Geometry check sheet. Reference: drawing and pictorial views, mm from the part's lowest x, y, z. Give positions to 0.01 mm unless a question says otherwise; leave off trailing zeros. Order: outer loops, then holes, each group sorted by start corner. A loop starts at its lowest first (then second) coordinate and runs counter-clockwise, first axis right, second up. Notation, with made-up numbers: (89.25, 88.5) -> (126.25, 88.5) arc R7 ccw to (126.25, 99.5) -> close; hole circle Ø5 at (-12, 81.5). An arc over 180 degrees is marked (long way). Write each question's results on one line, items separated by ' | '.
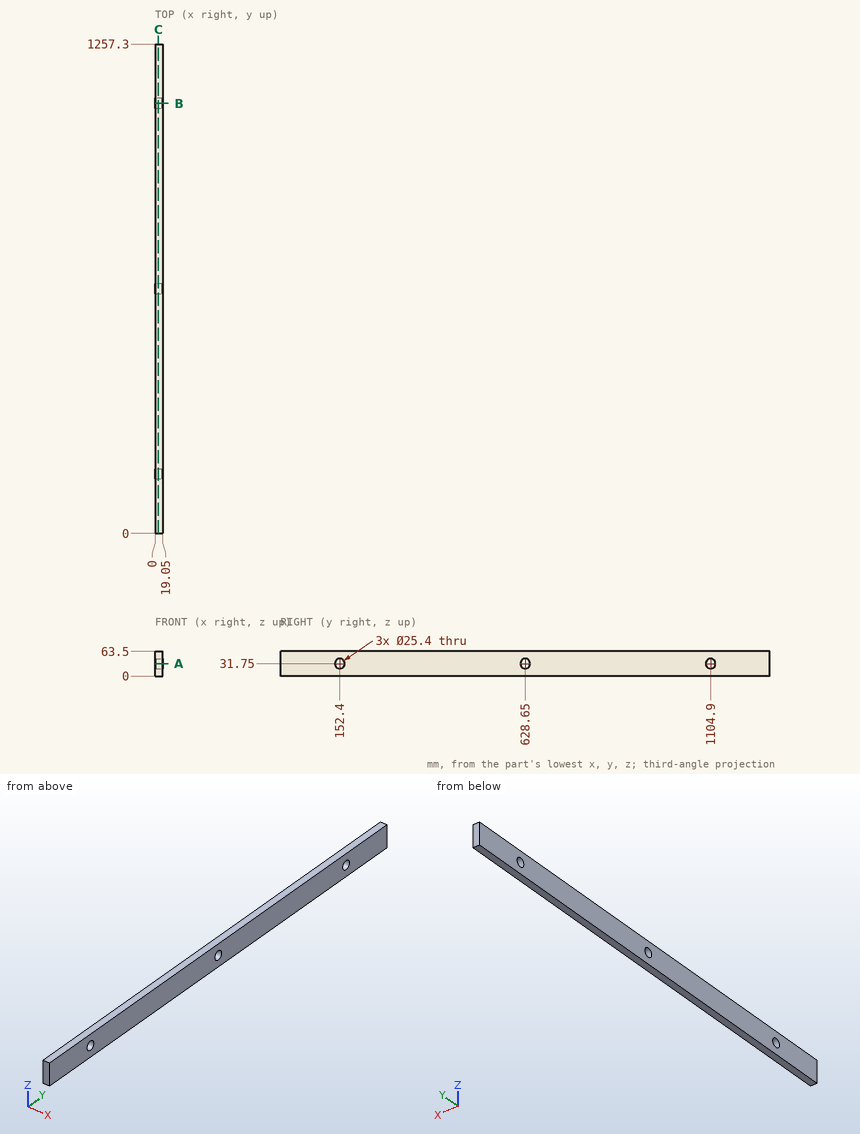
1. Material ranges on probe 1 along Z at (x, y) = (12.5, 628.65); probe 2 along Y at (x, z) = (10.25, 42); probe 3 along Y at (x, z) = (10.25, 43), recorded low to high. Write a range as from..to.
Verdict:
probe 1: z = 0..19.05, 44.45..63.5 | probe 2: y = 0..144.9, 159.9..621.15, 636.15..1097.4, 1112.4..1257.3 | probe 3: y = 0..146.51, 158.29..622.76, 634.54..1099.01, 1110.79..1257.3
2. Section check A-A on z = 31.75. Record the cut outline in (x, y).
Verdict:
outline: (0, 0) -> (19.05, 0) -> (19.05, 139.7) -> (0, 139.7) -> close; (0, 165.1) -> (19.05, 165.1) -> (19.05, 615.95) -> (0, 615.95) -> close; (0, 641.35) -> (19.05, 641.35) -> (19.05, 1092.2) -> (0, 1092.2) -> close; (0, 1117.6) -> (19.05, 1117.6) -> (19.05, 1257.3) -> (0, 1257.3) -> close
3. Gauge pin test, flat end, axial feed: pin 1 Ø15 at (y, z) = (152.4, 31.75) entering from +X. Record the tip position at first contact, or that the pin passes through.
Verdict:
pin 1: passes through
4. Section check B-B on y = 1104.9. Record the cut outline in (x, z).
Verdict:
outline: (0, 0) -> (19.05, 0) -> (19.05, 19.05) -> (0, 19.05) -> close; (0, 44.45) -> (19.05, 44.45) -> (19.05, 63.5) -> (0, 63.5) -> close
5. Section check C-C on x = 8.25. Record the cut outline in (y, z), then the cut area to 3 significant figures.
Verdict:
outline: (0, 0) -> (1257.3, 0) -> (1257.3, 63.5) -> (0, 63.5) -> close; hole circle Ø25.4 at (152.4, 31.75); hole circle Ø25.4 at (628.65, 31.75); hole circle Ø25.4 at (1104.9, 31.75) | area: 78,300 mm^2
